Verification items for the finished model (mm, model axes). Face numbers are marked on the shaded views. A direction names the side the tool comes from. Give positions to 0.01 mm unless a question says otherwise; leave off trailing zeros. Order: outer loops, then holes, each group sorted by start corner. A loop starts at its lowest first (then second) coordinate and runs counter-clockwise, first axis right, second up.
from build123d import *

# Parameters (mm, degrees)
SKETCH1_R           = 1.85
BOSS_EXTRUDE1_DEPTH = 3.1
SKETCH2_R           = 1.5
BOSS_EXTRUDE2_DEPTH = 1
SKETCH3_R           = 1.1
BOSS_EXTRUDE3_DEPTH = 2
SKETCH6_W           = 5
SKETCH6_H           = 5
BOSS_EXTRUDE4_DEPTH = 60
SKETCH7_R           = 1
CUT_EXTRUDE1_DEPTH  = 24


with BuildPart() as part:
    # Sketch1 → Boss-Extrude1 (new body)
    with BuildSketch(Plane(origin=(0, 0, 0), x_dir=(1, 0, 0), z_dir=(0, 1, 0))):
        with Locations(Location((0, 0, 0), (0, 0, 90))):
            Circle(SKETCH1_R)
    extrude(amount=BOSS_EXTRUDE1_DEPTH)

    # Sketch2 → Boss-Extrude2 (add)
    with BuildSketch(Plane(origin=(0, 3.1, 0), x_dir=(1, 0, 0), z_dir=(0, 1, 0))):
        with Locations(Location((0, 0, 0), (0, 0, 270))):
            Circle(SKETCH2_R)
    extrude(amount=BOSS_EXTRUDE2_DEPTH)

    # Sketch3 → Boss-Extrude3 (add)
    with BuildSketch(Plane(origin=(0, 4.1, 0), x_dir=(1, 0, 0), z_dir=(0, 1, 0))):
        with Locations(Location((0, 0, 0), (0, 0, 270))):
            Circle(SKETCH3_R)
    extrude(amount=BOSS_EXTRUDE3_DEPTH)

    # Loft1: read off the stored shape, not the designer's step
    # Loft1: loft between two sections, ruled curve by curve
    loft1_from = [
        Edge.make_bspline([(0, 6.1, 1.85), (3.7, 6.1, 1.85), (3.7, 6.1, -1.85), (0, 6.1, -1.85), (-3.7, 6.1, -1.85), (-3.7, 6.1, 1.85), (0, 6.1, 1.85)], [0, 0, 0, 0, 0.5, 0.5, 0.5, 1, 1, 1, 1], 3, [1, 0.333333333, 0.333333333, 1, 0.333333333, 0.333333333, 1]),
    ]
    loft1_to = [
        Edge.make_bspline([(0.620465421, 8.6, 0.968257539), (2.556980499, 8.6, -0.272673303), (1.316049657, 8.6, -2.209188381), (-0.620465421, 8.6, -0.968257539), (-2.556980499, 8.6, 0.272673303), (-1.316049657, 8.6, 2.209188381), (0.620465421, 8.6, 0.968257539)], [0, 0, 0, 0, 0.5, 0.5, 0.5, 1, 1, 1, 1], 3, [1, 0.333333333, 0.333333333, 1, 0.333333333, 0.333333333, 1]),
    ]
    loft1 = Solid(Shell([*[Face.make_surface_from_curves(loft1_from[k], loft1_to[k]) for k in range(1)], Face(Wire(loft1_from)), Face(Wire(loft1_to))]))
    add(loft1)

    # Sketch6 → Boss-Extrude4 (add)
    with BuildSketch(Plane.XZ):
        Rectangle(SKETCH6_W, SKETCH6_H)
    extrude(amount=BOSS_EXTRUDE4_DEPTH)

    # Sketch7 → Cut-Extrude1 (cut)
    with BuildSketch(Plane.XZ.offset(60)):
        with Locations(Location((0, 0, 0), (0, 0, 270))):
            Circle(SKETCH7_R)
    extrude(amount=-CUT_EXTRUDE1_DEPTH, mode=Mode.SUBTRACT)


solid = part.part
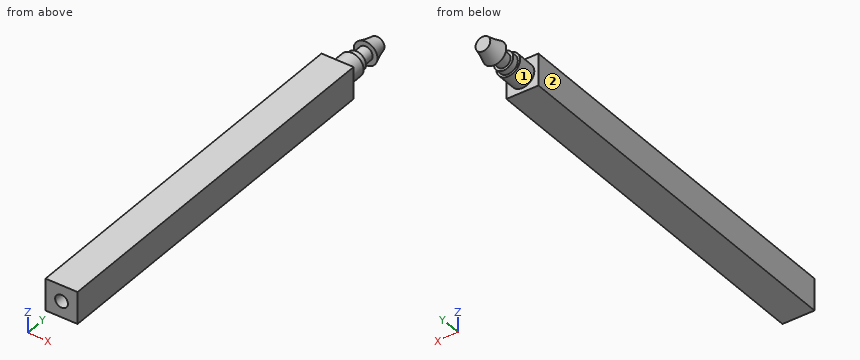
(1) Set-up check for the marked faces 1 and 2: record each of +Z, -Z, +X, -X, +Y, -Y from which the full face is reachable in a straight line by a thin tool's end or side.
Solved:
face 1: +Y
face 2: +Z, -Z, -X, +Y, -Y
(2) Section check A-A, the plane y = -39. Enter the section's corners in (x, z), then the cut area to 3 significant figures.
Solved:
outline: (-2.5, -2.5) - (2.5, -2.5) - (2.5, 2.5) - (-2.5, 2.5) - close; hole circle Ø2 at (0, 0)
area: 21.9 mm2
(3) Scan lines: line 1 (X direction, y = -44, z = 0); line 2 (Y direction, x = 0.05, z = 0.6); line 3 (Y direction, x = 1.6, z = -1.3). Record each from-to range of solid material in increasing order.
Solved:
line 1: x = -2.5 to -1, 1 to 2.5
line 2: y = -36 to 8.6
line 3: y = -60 to 0
